```python
from build123d import *

# Parameters (mm, degrees)
F1_DEPTH  = 76.454
F2_R      = 5.08
F3_R      = 12.5413462947
F3_R_2    = 8.7181007295
F3_R_3    = 8.2285725293
F4_DEPTH  = 25.4
F5_W      = 19.0680492669
F5_H      = 40.280263871
F6_DEPTH  = 9.144
F7_W      = 23.966927348
F7_H      = 13.4842246771
F8_DEPTH  = 3.048
F9_R      = 2.3003367046
F10_DEPTH = 5.334
F11_W     = 24.0274826065
F11_H     = 14.4164860249
F12_DEPTH = 8.128


with BuildPart() as f1:
    # F0 (on Top) → F1 (new body)
    with BuildSketch(Plane.XY):
        Polygon((-16.5632220721, -34.393885029), (16.5632220721, -34.393885029), (37.217222168, -8.4945880948), (29.8458948783, 23.8013069328), (0, 38.1743323818), (-29.8458948783, 23.8013069328), (-37.217222168, -8.4945880948), align=None)
    extrude(amount=F1_DEPTH)

    # F2
    f2_edges = [f1.edges().sort_by_distance(p)[0] for p in [
        (33.531559, 7.653359, 76.454),
        (14.922947, 30.98782, 76.454),
        (-14.922947, 30.98782, 76.454),
        (-33.531559, 7.653359, 76.454),
        (-26.890222, -21.444237, 76.454),
        (0, -34.393885, 76.454),
        (26.890222, -21.444237, 76.454),
        (29.845895, 23.801307, 38.227),
        (0, 38.174332, 38.227),
        (37.217222, -8.494588, 38.227),
        (16.563222, -34.393885, 38.227),
        (-29.845895, 23.801307, 38.227),
        (-37.217222, -8.494588, 38.227),
        (-16.563222, -34.393885, 38.227),
    ]]
    fillet(f2_edges, radius=F2_R)

    # F3 (on face) → F4 (join)
    with BuildSketch(Plane.XY.offset(76.454)):
        with Locations((-12.5352265313, 5.3862300701)):
            Circle(F3_R)
        with Locations((12.1435020119, 0)):
            Circle(F3_R_2)
        with Locations((-5.2882982418, -17.333868891)):
            Circle(F3_R_3)
    extrude(amount=F4_DEPTH)

    # F5 (on face) → F6 (join)
    with BuildSketch(Plane(origin=(33.5315585231, 7.653359419, 0), x_dir=(-0.222520934, 0.9749279122, 0), z_dir=(0.9749279122, 0.222520934, 0))):
        with Locations((1.0750833899, 20.1401319355)):
            Rectangle(F5_W, F5_H)
    extrude(amount=F6_DEPTH)

    # F7 (on face) → F8 (join)
    with BuildSketch(Plane(origin=(14.9229474392, 30.9878196573, 0), x_dir=(-0.9009688679, 0.4338837391, 0), z_dir=(0.4338837391, 0.9009688679, 0))):
        with Locations((2.1333593346, 58.0553635955)):
            Rectangle(F7_W, F7_H)
    extrude(amount=F8_DEPTH)

    # F9 (on face) → F10 (join)
    with BuildSketch(Plane(origin=(42.4462993521, 9.6880908391, 0), x_dir=(-0.222520934, 0.9749279122, 0), z_dir=(0.9749279122, 0.222520934, 0))):
        with Locations((3.9111254737, 19.3487424403)):
            Circle(F9_R)
    extrude(amount=-F10_DEPTH)

    # F11 (on face) → F12 (join)
    with BuildSketch(Plane.XZ.offset(34.393885029)):
        with Locations((-0.1144171692, 54.4746331871)):
            Rectangle(F11_W, F11_H)
    extrude(amount=F12_DEPTH)


solid = f1.part
```
Can you work these out from the model? Positions are in its coordinate system, mm. A direction names the side the tool comes from. Coordinates: 2 decimals unless noted, no trailing zeros. Loops run counter-clockwise (first coordinate to the right, second up) from the corner with the lowest first, then second, coordinate; pieces in that order, holes last. Notation, with made-up numbers: (36.25, 79) - (41.25, 79) arc R26 cw to (41.25, 108) - close; hole circle Ø8 at (31, 2.25). An arc over 180 degrees is marked (long way). Answer as CSV lines item,"result". Start each with the question number.
1) Suppose I cut it at B-B (z = 87). Please give me the cut outline in (x, y), plus the area to 3 significant figures.
2) Which directions (+Z, -Z, +X, -X, +Y, -Y) give clear straight access to the entire face, cutting with the end or side of a thin tool? Please do faces 1 (the flat face through (0, -38, 61.683)), 2 (the flat face through (-12.128, -38, 54)), 3 (the flat face through (24.45, 28.07, 57.96)).
3) Suppose I cut it at C-C (z = 46). Please give me the cut outline in (x, y).
4) I need wall thicknesses on line 1 (Z direction, x = 16.5, y = -26); line 2 (Y direction, x = -14, z = 40); line 3 (Y direction, x = -28, z = 29). Which ranges of each line are inside material? Lowest first, please. Write a range as from..to.
5) Thinking about a two-plate mould opening in Y: for faces 4 (the flat face through (38, 10, 40.28)), 5 (the cylindrical face through (0.198, -32.945, 74.926)), 6 (the flat face through (33.576, 7.461, 43.118)), which applies, pulls with the +Y half, pulls with the -Y half, needs draft (parallel to the pull), parting line crosses it, or undercut?
6) Suppose I cut it at D-D (z = 75). Please give me the cut outline in (x, y).
7) Suppose I cut it at A-A (z = 14.5). Please give me the cut outline in (x, y).
8) For pin 1 (6 mm diameter, centred on x = -13.5, y = -11.5, fed in from -Z); pin 2 (9 mm diameter, centred on y = -40, z = 56.5, fed in from +X); pin 3 (4 mm diameter, centred on x = 1, y = -37, fed in from -Z); pin 4 (2 mm diameter, centred on x = -27.5, z = 86, fed in from -Y), each with a flat end and sliding along its axis, tell me the tip position at first contact or that it passes through.
Check result:
1,outline,"circle Ø25.08 at (-12.54, 5.39); circle Ø16.46 at (-5.29, -17.33); circle Ø17.44 at (12.14, 0)"
1,area,"946 mm²"
2,face 1,"+Z, +X, -X, -Y"
2,face 2,"+Z, -Z, -X, -Y"
2,face 3,"+Z, -Z, +X"
3,outline,"(-36.67, -6.11) arc R5.08 ccw to (-35.69, -10.41) - (-18.09, -32.48) arc R5.08 ccw to (-14.12, -34.39) - (14.12, -34.39) arc R5.08 ccw to (18.09, -32.48) - (35.69, -10.41) arc R5.08 ccw to (36.67, -6.11) - (30.39, 21.42) arc R5.08 ccw to (27.64, 24.86) - (2.2, 37.11) arc R5.08 ccw to (-2.2, 37.11) - (-27.64, 24.86) arc R5.08 ccw to (-30.39, 21.42) - close"
4,line 1,"z = 0..76.45"
4,line 2,"y = -34.39..31.43"
4,line 3,"y = -20.05..24.67"
5,face 4,"needs draft"
5,face 5,"pulls with the -Y half"
5,face 6,"undercut"
6,outline,"(-35.19, -6.45) arc R3.56 ccw to (-34.5, -9.46) - (-16.9, -31.53) arc R3.56 ccw to (-14.12, -32.87) - (14.12, -32.87) arc R3.56 ccw to (16.9, -31.53) - (34.5, -9.46) arc R3.56 ccw to (35.19, -6.45) - (28.91, 21.08) arc R3.56 ccw to (26.98, 23.49) - (1.54, 35.74) arc R3.56 ccw to (-1.54, 35.74) - (-26.98, 23.49) arc R3.56 ccw to (-28.91, 21.08) - close"
7,outline,"(-36.67, -6.11) arc R5.08 ccw to (-35.69, -10.41) - (-18.09, -32.48) arc R5.08 ccw to (-14.12, -34.39) - (14.12, -34.39) arc R5.08 ccw to (18.09, -32.48) - (35.69, -10.41) arc R5.08 ccw to (36.67, -6.11) - (35.41, -0.59) - (44.33, 1.44) - (40.09, 20.03) - (31.17, 18) - (30.39, 21.42) arc R5.08 ccw to (27.64, 24.86) - (2.2, 37.11) arc R5.08 ccw to (-2.2, 37.11) - (-27.64, 24.86) arc R5.08 ccw to (-30.39, 21.42) - close"
8,pin 1,"stops at z = 0"
8,pin 2,"stops at x = 11.9"
8,pin 3,"stops at z = 47.27"
8,pin 4,"passes through"
